CAD build for the part. Positions are in the model's coordinates, mm. Face numbers are marked on the shaded views. A direction names the side the tool comes from. Coordinates: 2 decimals unless noted, no trailing zeros. Order: outer loops, then holes, each group sorted by start corner. A loop starts at its lowest first (then second) coordinate and runs counter-clockwise, first axis right, second up. Notation, with made-up numbers: M -19.5,69 L -0.5,69 A25 ccw -0.5,86 Z; hole C -12.75,7 d8. An arc over 180 degrees is marked long. Write item = value, one per line. Start each with the question number.
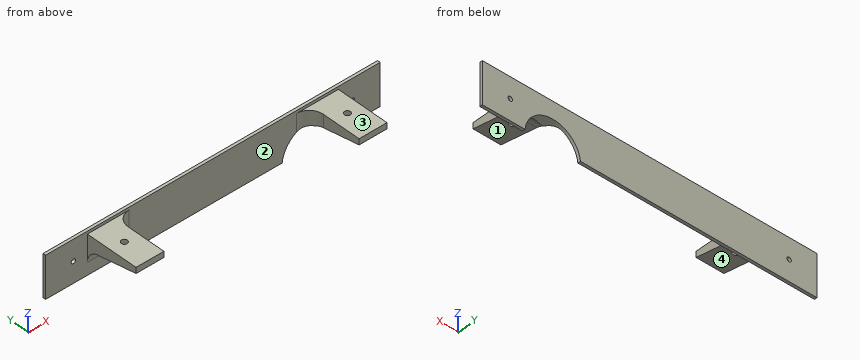
```python
from build123d import *

# Parameters (mm, degrees)
ESQUISSE1_W             = 240
ESQUISSE1_H             = 2
BOSS_EXTRU_1_DEPTH      = 30
ESQUISSE1_3_W           = 180
ESQUISSE1_3_H           = 38
BOSS_EXTRU_2_DEPTH      = 1.2
ESQUISSE2_R             = 1.6
ENL_V_MAT_EXTRU_1_DEPTH = 131
ESQUISSE3_W             = 180
ESQUISSE3_H             = 38
BOSS_EXTRU_3_DEPTH      = 10
ESQUISSE4_W             = 180
ESQUISSE4_H             = 38
ENL_V_MAT_EXTRU_2_DEPTH = 2
ESQUISSE5_W             = 140
ESQUISSE5_H             = 38
ENL_V_MAT_EXTRU_3_DEPTH = 130.247823966
CONG_1_R                = 10
CHANFREIN1_START        = -21.049758641
CHANFREIN1_DEPTH        = 8.142458431
ESQUISSE6_R             = 2.15
ENL_V_MAT_EXTRU_4_DEPTH = 130.247823996
ESQUISSE9_R             = 20
ENL_V_MAT_EXTRU_6_DEPTH = 10


with BuildPart() as part:
    # Esquisse1 → Boss.-Extru.1 (new body)
    with BuildSketch(Plane.XY):
        Rectangle(ESQUISSE1_W, ESQUISSE1_H)
    extrude(amount=-BOSS_EXTRU_1_DEPTH)

    # Esquisse1<3> → Boss.-Extru.2 (add)
    with BuildSketch(Plane.XY):
        with Locations((0, -20)):
            Rectangle(ESQUISSE1_3_W, ESQUISSE1_3_H)
    extrude(amount=-BOSS_EXTRU_2_DEPTH)

    # Esquisse2 → Enlèv. mat.-Extru.1 (cut, through all)
    with BuildSketch(Plane(origin=(0, 1, 0), x_dir=(1, 0, 0), z_dir=(0, 1, 0))):
        with Locations(Location((-100, 15, 0), (0, 0, 270))):
            Circle(ESQUISSE2_R)
        with Locations(Location((100, 15, 0), (0, 0, 270))):
            Circle(ESQUISSE2_R)
    extrude(amount=-ENL_V_MAT_EXTRU_1_DEPTH, mode=Mode.SUBTRACT)

    # Esquisse3 → Boss.-Extru.3 (add)
    with BuildSketch(Plane(origin=(0, 0, -1.2), x_dir=(-1, 0, 0), z_dir=(0, 0, -1))):
        with Locations((0, -20)):
            Rectangle(ESQUISSE3_W, ESQUISSE3_H)
    extrude(amount=BOSS_EXTRU_3_DEPTH)

    # Esquisse4 → Enlèv. mat.-Extru.2 (cut)
    with BuildSketch(Plane.XY):
        with Locations((0, -20)):
            Rectangle(ESQUISSE4_W, ESQUISSE4_H)
    extrude(amount=-ENL_V_MAT_EXTRU_2_DEPTH, mode=Mode.SUBTRACT)

    # Esquisse5 → Enlèv. mat.-Extru.3 (cut, through all)
    with BuildSketch(Plane.XY.offset(-2)):
        with Locations((0, -20)):
            Rectangle(ESQUISSE5_W, ESQUISSE5_H)
    extrude(amount=-ENL_V_MAT_EXTRU_3_DEPTH, mode=Mode.SUBTRACT)

    # Congé1
    cong_1_edges = [part.edges().sort_by_distance(p)[0] for p in [
        (-80, -1, -11.2),
        (80, -1, -11.2),
        (70, -1, -6.6),
        (-70, -1, -6.6),
    ]]
    fillet(cong_1_edges, radius=CONG_1_R)

    # Chanfrein1: read off the stored shape, not the designer's step
    # Chanfrein1 outline → Chanfrein1 (cut)
    with BuildSketch(Plane(origin=(0, 0, 0), x_dir=(1, 0, 0), z_dir=(0, 0.17430886736371906, 0.9846910270528403)).offset(CHANFREIN1_START)):
        with BuildLine():
            Line((-70, -37.321496906), (-70, -8.886181431))
            add(Edge.make_bspline(
                [(-69.997176769, -8.644881308), (-70, -8.765514336), (-70, -8.886181431)],
                knots=[4.688626138, 4.688626138, 4.688626138, 4.71238898, 4.71238898, 4.71238898], degree=2, weights=[1, 0.999929417, 1]))
            Line((-69.997176769, -8.644881308), (-90, -8.644881308))
            Line((-90, -8.644881308), (-90, -37.321496906))
            Line((-90, -37.321496906), (-70, -37.321496906))
        make_face()
        with BuildLine():
            Line((90, -37.321496906), (90, -8.644881308))
            Line((90, -8.644881308), (69.997176769, -8.644881308))
            add(Edge.make_bspline(
                [(70, -8.886181431), (70, -8.765514336), (69.997176769, -8.644881308)],
                knots=[1.570796327, 1.570796327, 1.570796327, 1.59455917, 1.59455917, 1.59455917], degree=2, weights=[1, 0.999929417, 1]))
            Line((70, -8.886181431), (70, -37.321496906))
            Line((70, -37.321496906), (90, -37.321496906))
        make_face()
    extrude(amount=CHANFREIN1_DEPTH, mode=Mode.SUBTRACT)

    # Esquisse6 → Enlèv. mat.-Extru.4 (cut, through all)
    with BuildSketch(Plane.XY.offset(-2)):
        with Locations((80, -19)):
            Circle(ESQUISSE6_R)
        with Locations((-80, -19)):
            Circle(ESQUISSE6_R)
    extrude(amount=-ENL_V_MAT_EXTRU_4_DEPTH, mode=Mode.SUBTRACT)

    # Esquisse9 → Enlèv. mat.-Extru.6 (cut)
    with BuildSketch(Plane(origin=(0, 1, 0), x_dir=(1, 0, 0), z_dir=(0, 1, 0))):
        with Locations((69.55, 32.2)):
            Circle(ESQUISSE9_R)
    extrude(amount=-ENL_V_MAT_EXTRU_6_DEPTH, mode=Mode.SUBTRACT)


solid = part.part
```
1. Mould opens along X. For the marked faces 1 and 2 say: released by +X, released by -X, zero draft, split by the parting line, or undercut.
2. Slice it at C-C (y = -19). Write the cut outline in (x, z).
3. 3-axis set-ups, long thin cutter, end or side, ignore diameter. For the marked faces 3 and 4: which of +Z, -Z, +X, -X, +Y, -Y reach the whole face in a straight line?
4. Probe L1, parallel to X at y = -19, z = -7; L2, parallel to Z at x = 100, y = 0.2; L3, parallel to Y at x = -98.5, z = -24.5. List the from-to ranges inside material, lowest first.
5. Slice it at D-D (x = -32). Write the cut outline in (y, z).
6. Flat gauge pins, fed straight in: pin 1 (15 mm diameter, centred on x = 80, y = -23, fed in from +Z); pin 2 (5 mm diameter, centred on x = -80, y = -19, fed in from -Z); pin 3 (15 mm diameter, centred on x = -44.5, z = -12.5, fed in from -Y); pin 4 (2 mm diameter, centred on y = -24.5, z = -11, fed in from +X). Where does each tip first touch, or does it go through?
7. Slice it at A-A (z = -26). Write the cut outline in (x, y), plus the area to 3 significant figures.
8. Slice it at B-B (y = -3.5). Write the cut outline in (x, z), plus the area to 3 significant figures.
Calculated:
q1.face_1 = zero draft
q1.face_2 = undercut
q2.outline = M -90,-9.74 L -82.15,-9.74 L -82.15,-2 L -90,-2 Z; M -77.85,-9.74 L -70,-9.74 L -70,-2 L -77.85,-2 Z; M 70,-9.74 L 77.85,-9.74 L 77.85,-2 L 70,-2 Z; M 82.15,-9.74 L 90,-9.74 L 90,-2 L 82.15,-2 Z
q3.face_3 = +Z, +X, -X, -Y
q3.face_4 = -Z, +X, -X, -Y
q4.L1 = -90 to -82.15, -77.85 to -70, 70 to 77.85, 82.15 to 90
q4.L2 = -30 to -16.6, -13.4 to 0
q4.L3 = -1 to 1
q5.outline = M -1,-30 L 1,-30 L 1,0 L -1,0 Z
q6.pin_1 = -2
q6.pin_2 = -10.19
q6.pin_3 = -1
q6.pin_4 = through
q7.outline = M -120,-1 L 50.54,-1 L 50.54,1 L -120,1 Z; M 88.56,-1 L 120,-1 L 120,1 L 88.56,1 Z
q7.area = 404 mm²
q8.outline = M -90,-14.59 L -66.61,-14.59 L -66.61,-2 L -90,-2 Z; M 66.61,-12.42 A20 cw 79.02,-14.59 L 90,-14.59 L 90,-2 L 66.61,-2 Z
q8.area = 567 mm²
